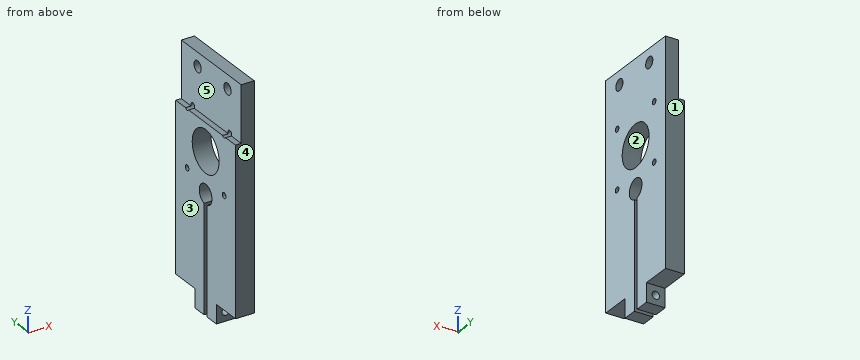
```python
from build123d import *

# Parameters (mm, degrees)
SKETCH_1_R          = 1.5
SKETCH_1_R_2        = 5.295460532
SKETCH_1_R_3        = 3
SKETCH_1_R_4        = 11.223257521
EXTRUDE_1_DEPTH     = 10
SKETCH_3_W          = 3
SKETCH_3_H          = 30
CUT_EXTRUDE_2_DEPTH = 50
CUT_EXTRUDE_3_DEPTH = 10
SKETCH_5_W          = 10
SKETCH_5_H          = 23.885605854
SKETCH_5_H_2        = 23.710254383
EXTRUDE_2_DEPTH     = 3
SKETCH_6_R          = 3.5
CUT_EXTRUDE_4_DEPTH = 5
SKETCH_7_R          = 2
CUT_EXTRUDE_5_DEPTH = 45
SKETCH_8_W          = 10
SKETCH_8_H          = 16
CUT_EXTRUDE_6_DEPTH = 10


with BuildPart() as part:
    # 草图1 → 凸台-拉伸1 (new body)
    with BuildSketch(Plane(origin=(66, 0, 0), x_dir=(0, 0, -1), z_dir=(1, 0, 0))):
        Polygon((48, 250), (-3, 250), (-17.702150009, 250), (-17.702150009, 300), (-3, 300), (48, 300), (108.216548797, 300), (108.216548797, 250), align=None)
        with Locations(Location((42.5, 259.5, 0), (0, 0, 90))):
            Circle(SKETCH_1_R, mode=Mode.SUBTRACT)
        with Locations(Location((42.5, 290.5, 0), (0, 0, 90))):
            Circle(SKETCH_1_R, mode=Mode.SUBTRACT)
        with Locations(Location((11.5, 259.5, 0), (0, 0, 90))):
            Circle(SKETCH_1_R, mode=Mode.SUBTRACT)
        with Locations(Location((11.5, 290.5, 0), (0, 0, 90))):
            Circle(SKETCH_1_R, mode=Mode.SUBTRACT)
        with Locations(Location((49, 275, 0), (0, 0, 90))):
            Circle(SKETCH_1_R_2, mode=Mode.SUBTRACT)
        with Locations(Location((-10.351075004, 286.4017148, 0), (0, 0, 90))):
            Circle(SKETCH_1_R_3, mode=Mode.SUBTRACT)
        with Locations(Location((-10.351075004, 261.4017148, 0), (0, 0, 90))):
            Circle(SKETCH_1_R_3, mode=Mode.SUBTRACT)
        with Locations(Location((27, 275, 0), (0, 0, 90))):
            Circle(SKETCH_1_R_4, mode=Mode.SUBTRACT)
    extrude(amount=EXTRUDE_1_DEPTH)

    # 草图3 → 切除-拉伸2 (cut)
    with BuildSketch(Plane.XZ.offset(-250)):
        with Locations((67.5, 2.702150009)):
            Rectangle(SKETCH_3_W, SKETCH_3_H)
    extrude(amount=-CUT_EXTRUDE_2_DEPTH, mode=Mode.SUBTRACT)

    # 草图4 → 切除-拉伸3 (cut)
    with BuildSketch(Plane(origin=(76, 0, 0), x_dir=(0, 0, -1), z_dir=(1, 0, 0))):
        Polygon((108.216548797, 276.289745617), (49.527425716, 276.289745617), (49.527425716, 273.885605854), (109.527425716, 273.885605854), (109.527425716, 276.289745617), align=None)
    extrude(amount=-CUT_EXTRUDE_3_DEPTH, mode=Mode.SUBTRACT)

    # 草图5 → 凸台-拉伸2 (add)
    with BuildSketch(Plane(origin=(0, 0, -108.216548797), x_dir=(-1, 0, 0), z_dir=(0, 0, -1))):
        with Locations((-71, 261.942802927)):
            Rectangle(SKETCH_5_W, SKETCH_5_H)
        with Locations((-71, 288.144872808)):
            Rectangle(SKETCH_5_W, SKETCH_5_H_2)
    extrude(amount=EXTRUDE_2_DEPTH)

    # 草图6 → 切除-拉伸4 (cut)
    with BuildSketch(Plane(origin=(0, 300, 0), x_dir=(1, 0, 0), z_dir=(0, 1, 0))):
        with Locations(Location((71, 106.216548797, 0), (0, 0, 180))):
            Circle(SKETCH_6_R)
    extrude(amount=-CUT_EXTRUDE_4_DEPTH, mode=Mode.SUBTRACT)

    # 草图7 → 切除-拉伸5 (cut)
    with BuildSketch(Plane(origin=(0, 295, 0), x_dir=(1, 0, 0), z_dir=(0, 1, 0))):
        with Locations(Location((71, 106.216548797, 0), (0, 0, 180))):
            Circle(SKETCH_7_R)
    extrude(amount=-CUT_EXTRUDE_5_DEPTH, mode=Mode.SUBTRACT)

    # 草图8 → 切除-拉伸6 (cut)
    with BuildSketch(Plane.ZY.offset(-66)):
        with Locations((-106.216548797, 292)):
            Rectangle(SKETCH_8_W, SKETCH_8_H)
        with Locations((-106.216548797, 258)):
            Rectangle(SKETCH_8_W, SKETCH_8_H)
    extrude(amount=-CUT_EXTRUDE_6_DEPTH, mode=Mode.SUBTRACT)


solid = part.part
```
CAD build for the part. Positions are in the model's coordinates, mm. Face numbers are marked on the shaded views. A direction names the side the tool comes from. Round coordinates to 2 decimals unless told otherwise and drop trailing zeros. Order: outer loops, then holes, each group sorted by start corner. A loop starts at its lowest first (then second) coordinate and runs counter-clockwise, first axis right, second up. Notation, with made-up numbers: (41.5, 79.5) - (74.5, 79.5) arc R11 cw to (74.5, 95.5) - close; hole circle Ø11 at (50, 27.25). An arc over 180 degrees is marked (long way). Answer in a Markdown table with one row per item. Add a question column.
(1) Mould opens along Y. For the marked faces 1, 2 and 3 say: +Y half, -Y half, draft (parallel to the pull), parting line (faces both ways), or undercut.
(2) Band-saw the part on C-C on z = -76.5. List the corners of the cut face in (x, y).
(3) Drop flat-ended pins along their axis: pin 1 Ø0.9 at (x, y) = (68, 294.5) entering from +Z; pin 2 Ø3 at (x, z) = (71.5, -108.5) entering from -Y; pin 3 Ø3 at (x, y) = (69, 254) entering from -Z. Give the stop position or say it passes through.
(4) 3-axis set-ups, long thin cutter, end or side, ignore diameter. For the marked faces 4 and 5: which of +Z, -Z, +X, -X, +Y, -Y reach the whole face in a straight line?
(5) Band-saw the part on B-B on x = 70.25. Count the separate pieces of the cut face and the enclosed holes in it, and give its area (3 significant figures).
(6) Band-saw the part on A-A on z = -42.5. List the corners of the cut face in (x, y), and give its area (3 significant figures).
(7) Probe L1, parallel to Y at x = 69.25, z = -11.5; L2, parallel to Z at x = 71.75, y = 275; L3, parallel to Y at x = 69.75, z = -54.5. List the from-to ranges inside material, lowest first. Write a range as [from, to].
(8) Band-saw the part on D-D on y = 293.5. List the corners of the cut face in (x, z).
Data:
| question | item | result |
|---|---|---|
| 1 | face 1 | +Y half |
| 1 | face 2 | undercut |
| 1 | face 3 | draft |
| 2 | outline | (66, 250) - (76, 250) - (76, 273.89) - (66, 273.89) - close; (66, 276.29) - (76, 276.29) - (76, 300) - (66, 300) - close |
| 3 | pin 1 | stops at z = -12.3 |
| 3 | pin 2 | stops at y = 266 |
| 3 | pin 3 | stops at z = -101.22 |
| 4 | face 4 | +Z, -Z, +X, -X, -Y |
| 4 | face 5 | +Z, -X, +Y, -Y |
| 5 | separate pieces | 3 |
| 5 | enclosed holes | 7 |
| 5 | area | 5,360 mm^2 |
| 6 | outline | (66, 250) - (76, 250) - (76, 258) - (66, 258) - close; (66, 261) - (76, 261) - (76, 289) - (66, 289) - close; (66, 292) - (76, 292) - (76, 300) - (66, 300) - close |
| 6 | area | 440 mm^2 |
| 7 | L1 | y = [250, 258], [261, 289], [292, 300] |
| 7 | L2 | z = [-43.7, -38.22], [-15.78, 17.7] |
| 7 | L3 | y = [250, 273.89], [276.29, 300] |
| 8 | outline | (66, -101.22) - (76, -101.22) - (76, 17.7) - (69, 17.7) - (69, -12.3) - (66, -12.3) - close |
